The listing builds one solid part. Answer for the finished solid, in the listing's coordinates (mm). A direction names the side the tool comes from. Give positions to 0.01 mm unless a question says otherwise; leave off trailing zeros. Loops run counter-clockwise (first coordinate to the right, second up) from the corner with the lowest first, then second, coordinate; pieces in that order, holes last. Notation, with made-up numbers: M -27,37 L 23,37 A21 ccw 23,53 Z; hole C -7,-13.75 d9. An arc over 180 degrees is marked long. Use one line per item in the form item = value. Start each with the question number.
1. Each of these flat-tipped pins is pushed along its axis until it touches: pin 1 Ø3 at (x, y) = (1.5, 50.5) entering from +Z; pin 2 Ø2 at (y, z) = (-8, 4.5) entering from -X; pin 3 Ø1 at (y, z) = (-6.5, 4) entering from +X; pin 4 Ø2.5 at (x, y) = (-50.15, 0) entering from +Z. Where does it stop, or does it pass through?
2. The part is cut by section B-B (z = 6.75). Give the number of separate pieces and of enclosed holes in the cut face, and give its area (3 significant figures).
3. For faces 1 (the face through (52, -1, 4)), 2 (the face through (0.761, 48.686, 1.972)), determine the directions among +Z, -Z, +X, -X, +Y, -Y from which every point of the face is accessible in a straight line to the end or side of a thin tool.
4. The mould has two halves that part along Y. Classify faces 3 (the face through (-51.8, 0.07, 1.97)), 4 (the face through (-15, -43, 0)): released by +Y, released by -Y, zero draft, split by the parting line, or undercut.
5. The part is cut by section A-A (y = 0). Write down the section's boundary in (x, z).
6. Straight lines are drawn through the part: line 1 (Y direction, x = 0, z = 2.8); line 2 (Y direction, x = 36.5, z = 5.5); line 3 (X direction, y = -38, z = 9) (3 decimals). For each, find the intervals that lie inside material, in ascending order. Write a range as from..to.
from build123d import *

# Parameters (mm, degrees)
SKETCH1_R           = 65.3
SKETCH1_R_2         = 45.3
SKETCH1_R_3         = 1.65
BOSS_EXTRUDE1_DEPTH = 10
FILLET1_R           = 5
SKETCH2_R           = 3.25
CUT_EXTRUDE1_DEPTH  = 6


with BuildPart() as part:
    # Sketch1 → Boss-Extrude1 (new body)
    with BuildSketch(Plane.XY):
        Circle(SKETCH1_R)
        Circle(SKETCH1_R_2, mode=Mode.SUBTRACT)
        with Locations((35.461405077, -35.461405077)):
            Circle(SKETCH1_R_3, mode=Mode.SUBTRACT)
        with Locations((0, -50.15)):
            Circle(SKETCH1_R_3, mode=Mode.SUBTRACT)
        with Locations((-35.461405077, -35.461405077)):
            Circle(SKETCH1_R_3, mode=Mode.SUBTRACT)
        with Locations((-50.15, 0)):
            Circle(SKETCH1_R_3, mode=Mode.SUBTRACT)
        with Locations((-35.461405077, 35.461405077)):
            Circle(SKETCH1_R_3, mode=Mode.SUBTRACT)
        with Locations((0, 50.15)):
            Circle(SKETCH1_R_3, mode=Mode.SUBTRACT)
        with Locations((35.461405077, 35.461405077)):
            Circle(SKETCH1_R_3, mode=Mode.SUBTRACT)
        with Locations((50.15, 0)):
            Circle(SKETCH1_R_3, mode=Mode.SUBTRACT)
    extrude(amount=BOSS_EXTRUDE1_DEPTH)

    # Fillet1
    fillet1_edges = [part.edges().sort_by_distance(p)[0] for p in [
        (-65.3, 0, 10),
    ]]
    fillet(fillet1_edges, radius=FILLET1_R)

    # Sketch2 → Cut-Extrude1 (cut)
    with BuildSketch(Plane.XY.offset(10)):
        with Locations((-50.15, 0)):
            Circle(SKETCH2_R)
        with Locations((-35.461405077, -35.461405077)):
            Circle(SKETCH2_R)
        with Locations((-35.461405077, 35.461405077)):
            Circle(SKETCH2_R)
        with Locations((0, 50.15)):
            Circle(SKETCH2_R)
        with Locations((35.461405077, 35.461405077)):
            Circle(SKETCH2_R)
        with Locations((50.15, 0)):
            Circle(SKETCH2_R)
        with Locations((35.461405077, -35.461405077)):
            Circle(SKETCH2_R)
        with Locations((0, -50.15)):
            Circle(SKETCH2_R)
    extrude(amount=-CUT_EXTRUDE1_DEPTH, mode=Mode.SUBTRACT)


solid = part.part
Derived:
q1.pin_1 = 4
q1.pin_2 = -64.92
q1.pin_3 = 65.02
q1.pin_4 = through
q2.separate_pieces = 1
q2.enclosed_holes = 9
q2.area = 6,550 mm2
q3.face_1 = +Z
q3.face_2 = +Z, -Z
q4.face_3 = undercut
q4.face_4 = zero draft
q5.outline = M -65.3,0 L -51.8,0 L -51.8,4 L -53.4,4 L -53.4,10 L -60.3,10 A5 ccw -65.3,5 Z; M -48.5,0 L -45.3,0 L -45.3,10 L -46.9,10 L -46.9,4 L -48.5,4 Z; M 45.3,0 L 48.5,0 L 48.5,4 L 46.9,4 L 46.9,10 L 45.3,10 Z; M 51.8,0 L 65.3,0 L 65.3,5 A5 ccw 60.3,10 L 53.4,10 L 53.4,4 L 51.8,4 Z
q6.line_1 = -65.3..-51.8, -48.5..-45.3, 45.3..48.5, 51.8..65.3
q6.line_2 = -54.12..-38.54, -32.38..-26.83, 26.83..32.38, 38.54..54.12
q6.line_3 = -50.625..-37.491, -33.432..-24.659, 24.659..33.432, 37.491..50.625
